For this review, take the finished solid that the model builds, in its own axes (mm). A direction names the side the tool comes from. Coordinates: 2 decimals unless noted, no trailing zeros. Loops run counter-clockwise (first coordinate to the right, second up) from the corner with the lowest first, then second, coordinate; pieces in that order, holes last. Notation, with made-up numbers: (71, 65) - (123, 65) arc R34 cw to (123, 99) - close; hole circle Ø6 at (46, 3). An arc over 180 degrees is marked (long way). One line per item, written item: value. Start each with the question number.
1. Take a section at A-A, the plane x = 29.5. State the section outline as (y, z) points, and give its area (3 significant figures).
2. For faces 5 (the face through (-75.701, 8, 7)), 6 (the face through (72.299, -8, 4)), 7 (the face through (-75.701, -24, 2)), 8 (the face through (62.299, 9, 2)), 9 (the face through (62.299, -24, 1)), list the 3-axis set-ups (+Z, -Z, +X, -X, +Y, -Y) from which the entire face can be reached by the end or side of a thin tool; tool diameter is ignored.
3. Take a section at B-B, the plane z = 6.75. State the section outline as (x, y) points.
4. The part is to be moulded in two halves that separate along Z. For faces 1 (the face through (-81, 7.317, 4)), 2 (the face through (-7.67, -24.71, 6.03)), 3 (the face through (-8, -7, 8)), 4 (the face through (-7.67, -24.65, 2.03)), say which applies: released by +Z, released by -Z, zero draft, split by the parting line, or undercut.
5. To check wall thickness, follow line 1 (X direction, y = 8.5, z = 1); line 2 (Y direction, x = -57.5, z = 3.75); line 3 (Y direction, x = 63, z = 2.5). State the ranges of each line that lie inside material, in increasing order. Write a range as from..to.
6. Insertion check: pin 1 (4.5 mm diameter, centred on y = -24, z = 2, fed in from +X); pin 2 (3 mm diameter, centred on y = -25.5, z = 6.5, fed in from +X); pin 3 (3 mm diameter, centred on y = -25, z = 5.5, fed in from -X); pin 4 (4 mm diameter, centred on x = 68.5, z = 5, fed in from -Y). Each pin has a flat end and moves straight along its axis. Give the tip position at first contact, or say it passes through.
```python
from build123d import *

# Parameters (mm, degrees)
F1_DEPTH = 8
F4_DEPTH = 148.001


with BuildPart() as f1:
    # F0 (on Top) → F1 (new body)
    with BuildSketch(Plane.XY):
        Polygon((-75.700524, 7.317285), (-85.700524, 7.317285), (-85.700524, -22.682715), (-75.700524, -22.682715), (-75.700524, -26.682715), (62.299476, -26.682715), (62.299476, -22.682715), (72.299476, -22.682715), (72.299476, 7.317285), (62.299476, 7.317285), (62.299476, 11.317285), (-75.700524, 11.317285), align=None)
    extrude(amount=F1_DEPTH)

    # F2 (on face) + F3 (on face) → F4 (cut, through all)
    with BuildSketch(Plane(origin=(-75.700524, 0, 0), x_dir=(0, -1, 0), z_dir=(-1, 0, 0))):
        Polygon((22.682715, 4), (26.682715, 0), (26.682715, 8), align=None)
    with BuildSketch(Plane(origin=(-75.700524, 0, 0), x_dir=(0, -1, 0), z_dir=(-1, 0, 0))):
        Polygon((-7.317285, 4), (-11.317285, 8), (-11.317285, 0), align=None)
    extrude(amount=-F4_DEPTH, mode=Mode.SUBTRACT)


solid = f1.part
```
Solutions:
1. outline: (-26.68, 0) - (11.32, 0) - (7.32, 4) - (11.32, 8) - (-26.68, 8) - (-22.68, 4) - close
1. area: 272 mm2
2. face 5: +Z, -Z, -X, +Y
2. face 6: +Z, -Z, +X, +Y, -Y
2. face 7: +Z, -Z, -X, -Y
2. face 8: +Z, -Z, +X, +Y
2. face 9: +Z, -Z, +X, -Y
3. outline: (-85.7, -22.68) - (-75.7, -22.68) - (-75.7, -25.43) - (62.3, -25.43) - (62.3, -22.68) - (72.3, -22.68) - (72.3, 7.32) - (62.3, 7.32) - (62.3, 10.07) - (-75.7, 10.07) - (-75.7, 7.32) - (-85.7, 7.32) - close
4. face 1: zero draft
4. face 2: undercut
4. face 3: released by +Z
4. face 4: undercut
5. line 1: -75.7..62.3
5. line 2: -22.93..7.57
5. line 3: -22.68..7.32
6. pin 1: x = 72.3
6. pin 2: x = 62.3
6. pin 3: x = -75.7
6. pin 4: y = -22.68
